Drawing for the job (mm, zero at the part's lowest x, y, z). Coordinates: 2 decimals unless noted, no trailing zeros. Write each loop counter-clockwise with the first axis right and the second up, starting at its lowest first coordinate (ties: lowest second). Pieces come first, ordered by that corner, then holes. Notation, with made-up numbers: (68, -9) - (87, -9) arc R19 cw to (87, 27) - close; hole circle Ø6 at (37.25, 11.5). An arc over 180 degrees is marked (long way). Write each question's results on one line, items separated by ' | '.
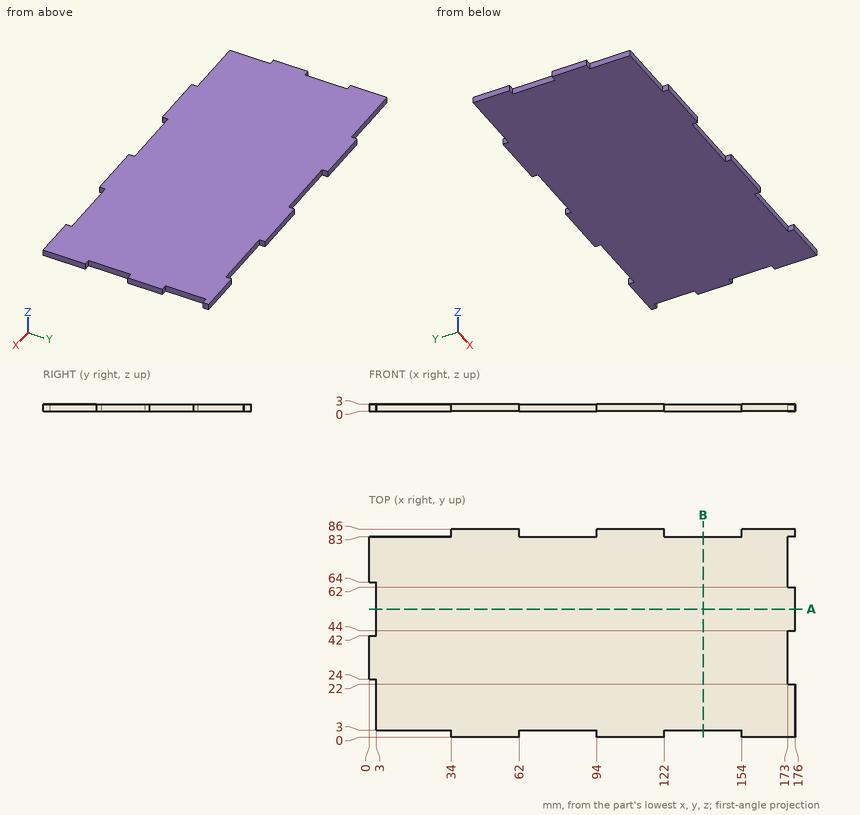
(1) Flat gauge pins, fed straight in: P1, Ø1.5, axis at x = 143.5, z = 2, coming from the +Y side; P2, Ø0.9, axis at y = 58, z = 2, coming from the -X side; P3, Ø1.5, axis at y = 38, z = 1, coming from the +X side; P4, Ø1, axis at y = 37.5, z = 1.5, coming from the -X side. Where does each tip first touch, or does it go through?
Return value:
P1: stops at y = 83 | P2: stops at x = 3 | P3: stops at x = 173 | P4: stops at x = 0
(2) Saw through at A-A on y = 53. Write the cut outline in (x, z).
Return value:
outline: (3, 0) - (176, 0) - (176, 3) - (3, 3) - close
(3) Saw through at B-B on x = 138. Write the cut outline in (y, z), then the cut area to 3 significant figures.
Return value:
outline: (3, 0) - (83, 0) - (83, 3) - (3, 3) - close | area: 240 mm^2
(4) Wall check: line 1 (X direction, y = 8.5, z = 0.25); line 2 (X direction, y = 78, z = 1.5); line 3 (Y direction, x = 84, z = 0.8). Give the ranges that are in metal, low to high. Write a range as from..to.
Return value:
line 1: x = 3..176 | line 2: x = 0..173 | line 3: y = 3..83
